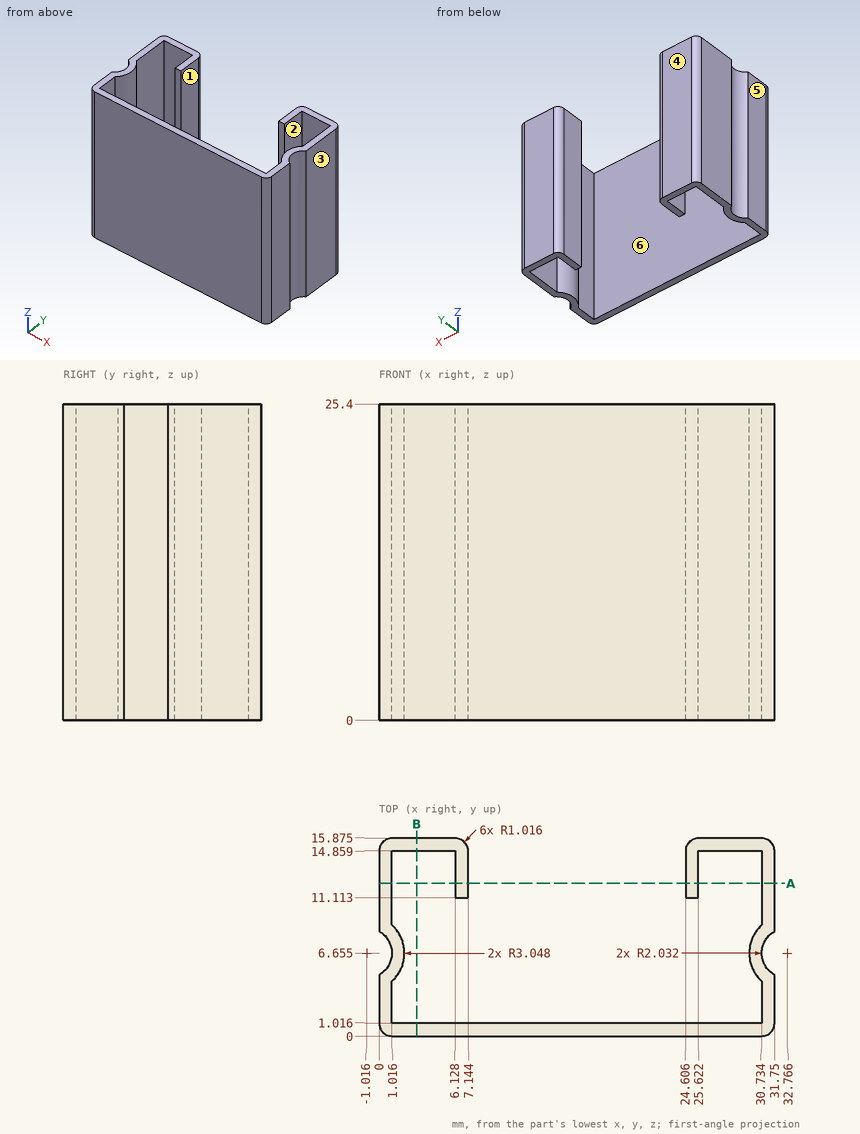
Could you check a few things on this drawing? It's one solid part, dimensions in mm from its lowest x, y, z. A direction names the side the tool comes from. Coordinates: 2 decimals unless noted, no trailing zeros. Write each loop counter-clockwise with the first axis right and the second up, starting at its lowest first coordinate (ties: lowest second). Pieces come first, ordered by that corner, then holes. Notation, with made-up numbers: (43, 43.25) - (64, 43.25) arc R14 cw to (64, 68.25) - close; hole circle Ø3 at (-8, 1.25). An arc over 180 degrees is marked (long way). Return JSON: item names as keys, results as strings. Group by question number.
Item 1: I'm going to push flat-ended pins straight in: pin 1 Ø3 at (x, z) = (12, 14.5) entering from +Y; pin 2 Ø5 at (x, y) = (27.5, 9) entering from +Z. Where does each tip first touch, or does it pass through?
Item 2: If we section it at A-A (y = 12.25): Count the separate pieces of the cut face and the enclosed holes in it, then the cut area to 3 significant figures.
Item 3: Please list where these lines run through material, in increasing order: probe 1 along Y at (x, z) = (29, 18.75) (1 decimal); probe 2 along Y at (x, z) = (30, 17.25) (1 decimal); probe 3 along Y at (x, z) = (14, 16.25) (1 decimal).
Item 4: Which directions (+Z, -Z, +X, -X, +Y, -Y) give clear straight access to the entire face, cutting with the end or side of a thin tool? Please do the marked faces 1, 2 and 3.
Item 5: We'd pull the mould along Y, two halves only. Please class the marked faces 4, 5 and 6: pulls with the +Y half, pulls with the -Y half, needs draft (parallel to the pull), parting line crosses it, or undercut.
Item 6: If we section it at B-B (x = 3): Write out the boundary of the cut face in (y, z) (1 decimal).
Return value:
{
 "1": {"pin 1": "stops at y = 1.02", "pin 2": "passes through"},
 "2": {"separate pieces": "4", "enclosed holes": "0", "area": "103 mm^2"},
 "3": {"probe 1": "y = 0 to 1, 14.9 to 15.9", "probe 2": "y = 0 to 1, 5.4 to 7.9, 14.9 to 15.9", "probe 3": "y = 0 to 1"},
 "4": {"face 1": "+Z, -Z, +Y", "face 2": "+Z, -Z", "face 3": "+Z, -Z, +X, +Y, -Y"},
 "5": {"face 4": "pulls with the +Y half", "face 5": "needs draft", "face 6": "undercut"},
 "6": {"outline": "(0, 0) - (1, 0) - (1, 25.4) - (0, 25.4) - close; (14.9, 0) - (15.9, 0) - (15.9, 25.4) - (14.9, 25.4) - close"}
}
